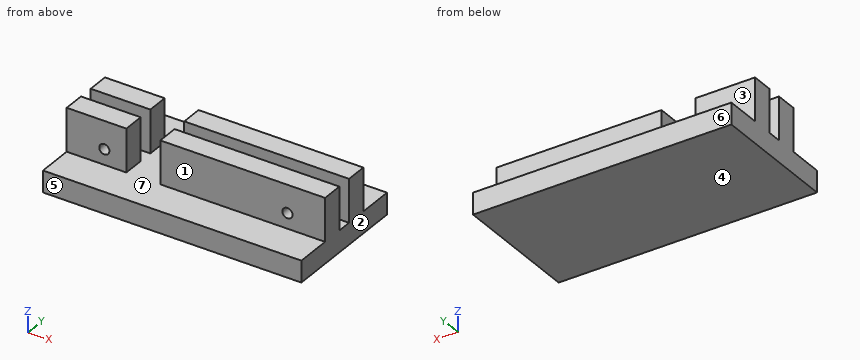
```python
from build123d import *

# Parameters (mm, degrees)
F0_W     = 76.2
F0_H     = 38.1
F1_DEPTH = 6.35
F2_W     = 6.35
F2_H     = 19.05
F3_DEPTH = 76.2
F4_R     = 1.5
F4_W     = 10
F4_H     = 12.7
F5_DEPTH = 17.018


with BuildPart() as f1:
    # F0 (on Top) → F1 (new body)
    with BuildSketch(Plane.XY):
        Rectangle(F0_W, F0_H)
    extrude(amount=F1_DEPTH)

    # F2 (on face) → F3 (join, through all)
    with BuildSketch(Plane.YZ.offset(38.1)):
        with Locations((-5.334, 9.525)):
            Rectangle(F2_W, F2_H)
        with Locations((5.334, 9.525)):
            Rectangle(F2_W, F2_H)
    extrude(amount=-F3_DEPTH)

    # F4 (on face) → F5 (cut, through all)
    with BuildSketch(Plane.XZ.offset(8.509)):
        with Locations((-27, 10.85)):
            Circle(F4_R)
        with Locations((27, 10.85)):
            Circle(F4_R)
        with Locations((-15.5, 12.7)):
            Rectangle(F4_W, F4_H)
    extrude(amount=-F5_DEPTH, mode=Mode.SUBTRACT)


solid = f1.part
```
Geometry check sheet. Reference: the model listing, model coordinates, mm. Face numbers are marked on the shaded views. A direction names the side the tool comes from. Coordinates: 2 decimals unless noted, no trailing zeros. Loops run counter-clockwise (first coordinate to the right, second up) from the corner with the lowest first, then second, coordinate; pieces in that order, holes last.
Item 1: Sectioned sample at C-C, the plane y = -7. Record the boundary of the cut face in (x, z), then the cut area to 3 significant figures.
Item 2: Sectioned sample at D-D, the plane x = -22. Record the boundary of the cut face in (y, z).
Item 3: Go/stop test with flat-tipped pins: pin 1 Ø4 at (x, z) = (11.5, 13) entering from -Y; pin 2 Ø4 at (x, z) = (15, 12) entering from +Y. Record where each tip stops, or that it passes through.
Item 4: Sectioned sample at A-A, the plane x = 27. Record the boundary of the cut face in (y, z), then the cut area to 3 significant figures.
Item 5: Sectioned sample at B-B, the plane z = 10.85. Count the separate pieces of the cut face and the enclosed holes in it, then the cut area to 3 significant figures.
Item 6: Release check for a two-part mould opening along Y. For the marked faces 4, 5, 6 and 7 record: released by +Y, released by -Y, zero draft, split by the parting line, or undercut.
Item 7: Access from +Z, -Z, +X, -X, +Y, -Y to the whole of each face (thin tool, end or side, straight path). Record for the marked faces 1, 2 and 3.
Item 8: Thickness scan on line 1 (Y direction, x = 22.5, z = 15.5); line 2 (X direction, y = -6, z = 11.25); line 3 (Z direction, x = -27, y = 4). Record the ranges inside material, lowest first.
Check result:
1. outline: (-38.1, 0) - (38.1, 0) - (38.1, 19.05) - (-10.5, 19.05) - (-10.5, 6.35) - (-20.5, 6.35) - (-20.5, 19.05) - (-38.1, 19.05) - close; hole circle Ø3 at (-27, 10.85); hole circle Ø3 at (27, 10.85)
1. area: 1,310 mm2
2. outline: (-19.05, 0) - (19.05, 0) - (19.05, 6.35) - (8.51, 6.35) - (8.51, 19.05) - (2.16, 19.05) - (2.16, 6.35) - (-2.16, 6.35) - (-2.16, 19.05) - (-8.51, 19.05) - (-8.51, 6.35) - (-19.05, 6.35) - close
3. pin 1: stops at y = -8.51
3. pin 2: stops at y = 8.51
4. outline: (-19.05, 0) - (19.05, 0) - (19.05, 6.35) - (8.51, 6.35) - (8.51, 9.35) - (2.16, 9.35) - (2.16, 6.35) - (-2.16, 6.35) - (-2.16, 9.35) - (-8.51, 9.35) - (-8.51, 6.35) - (-19.05, 6.35) - close; (-8.51, 12.35) - (-2.16, 12.35) - (-2.16, 19.05) - (-8.51, 19.05) - close; (2.16, 12.35) - (8.51, 12.35) - (8.51, 19.05) - (2.16, 19.05) - close
4. area: 365 mm2
5. separate pieces: 8
5. enclosed holes: 0
5. area: 765 mm2
6. face 4: zero draft
6. face 5: released by -Y
6. face 6: released by +Y
6. face 7: undercut
7. face 1: +Z, +X, -X, -Y
7. face 2: +Z, -Z, +X, +Y, -Y
7. face 3: +Z, +X, -X, +Y
8. line 1: y = -8.51 to -2.16, 2.16 to 8.51
8. line 2: x = -38.1 to -28.45, -25.55 to -20.5, -10.5 to 25.55, 28.45 to 38.1
8. line 3: z = 0 to 9.35, 12.35 to 19.05
